Design review of the part built by this model. Coordinates are the model's own, in mm. Coordinates: 2 decimals unless noted, no trailing zeros. Write each loop counter-clockwise with the first axis right and the second up, starting at its lowest first coordinate (ties: lowest second). Pieces come first, ordered by that corner, then holes.
Q1. For probe 1 along X at (y, z) = (8.75, -44.45); probe 2 along Z at (x, y) = (67.5, 9.5), list the stretches that pass through material, from the lowest coordinate up.
Q2. Take a section at A-A (z = -44.45). Give the boundary of the cut face in (x, y), and give its area (3 significant figures).
Q3. Take a section at B-B (x = 58.5). Give the boundary of the cut face in (y, z), and give its area (3 significant figures).
```python
from build123d import *

# Parameters (mm, degrees)
SKETCH1_W           = 127
SKETCH1_H           = 88.9
SKETCH1_R           = 14.2875
BOSS_EXTRUDE1_DEPTH = 11.90625
SKETCH2_W           = 127
SKETCH2_H           = 82.55
BOSS_EXTRUDE2_DEPTH = 11.90625


with BuildPart() as part:
    # Sketch1 → Boss-Extrude1 (new body)
    with BuildSketch(Plane(origin=(0, 0, 0), x_dir=(1, 0, 0), z_dir=(0, 1, 0))):
        with Locations((63.5, 44.45)):
            Rectangle(SKETCH1_W, SKETCH1_H)
        with Locations(Location((63.5, 44.45, 0), (0, 0, 270))):
            Circle(SKETCH1_R, mode=Mode.SUBTRACT)
    extrude(amount=BOSS_EXTRUDE1_DEPTH)

    # Sketch2 → Boss-Extrude2 (add)
    with BuildSketch(Plane(origin=(0, 11.90625, 0), x_dir=(1, 0, 0), z_dir=(0, 1, 0))):
        with Locations((63.5, 130.175)):
            Rectangle(SKETCH2_W, SKETCH2_H)
        with Locations((63.5, -41.275)):
            Rectangle(SKETCH2_W, SKETCH2_H)
    extrude(amount=-BOSS_EXTRUDE2_DEPTH)


solid = part.part
```
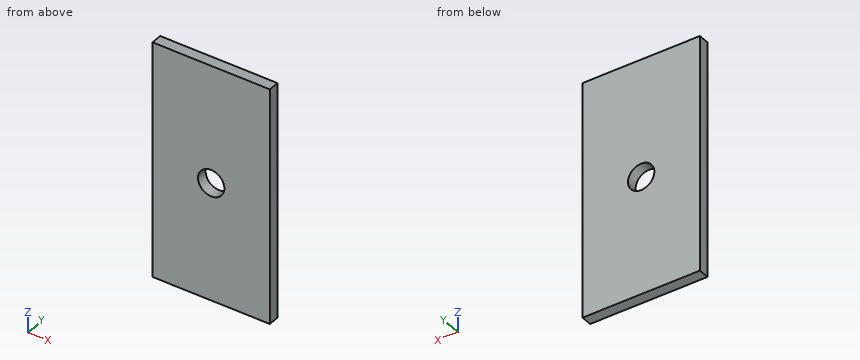
Response:
1. probe 1: x = 0 to 49.21, 77.79 to 127
1. probe 2: z = -171.45 to -58.17, -30.73 to 82.55
2. outline: (0, 0) - (49.21, 0) - (49.21, 11.91) - (0, 11.91) - close; (77.79, 0) - (127, 0) - (127, 11.91) - (77.79, 11.91) - close
2. area: 1,170 mm2
3. outline: (0, -171.45) - (11.91, -171.45) - (11.91, -57.83) - (0, -57.83) - close; (0, -31.07) - (11.91, -31.07) - (11.91, 82.55) - (0, 82.55) - close
3. area: 2,710 mm2
